```python
from build123d import *

# Parameters (mm, degrees)
F0_R      = 1.1
F1_DEPTH  = 4.75
F2_R      = 5
F3_DEPTH  = 5
F5_R      = 2
F7_DEPTH  = 0.8
F8_R      = 0.75
F9_R      = 9.5
F10_DEPTH = 3
F12_R     = 4.5172071506
F12_R_2   = 2.2672071506
F13_DEPTH = 3.7
F14_R     = 0.625
F15_DEPTH = 2
F16_SIZE  = 0.35


# Not quite as in the source:
# - a feature names something its author has since deleted; it is built from what else it names


with BuildPart() as f1:
    # F0 (on Top) → F1 (new body)
    with BuildSketch(Plane.XY):
        with BuildLine():
            Line((-5.0334316447, -3.2656646917), (-9.6784130262, -7.9106460732))
            ThreePointArc((-9.6784130262, -7.9106460732), (-7.1490584463, -10.2538267653), (-4.0757746589, -11.8168549509))
            ThreePointArc((-4.0757746589, -11.8168549509), (-3.593311946, -12.8676823003), (-2.8459674038, -13.75))
            Line((-2.8459674038, -13.75), (2.8459674038, -13.75))
            ThreePointArc((2.8459674038, -13.75), (3.593311946, -12.8676823003), (4.0757746589, -11.8168549509))
            ThreePointArc((4.0757746589, -11.8168549509), (7.1490584463, -10.2538267653), (9.6784130262, -7.9106460732))
            Line((9.6784130262, -7.9106460732), (5.0334316447, -3.2656646917))
            ThreePointArc((5.0334316447, -3.2656646917), (0, 6), (-5.0334316447, -3.2656646917))
        make_face()
        with Locations((0, -11.25)):
            Circle(F0_R, mode=Mode.SUBTRACT)
        with BuildLine():
            Line((-5.061459087, -6.82922604), (-3.2656646917, -5.0334316447))
            ThreePointArc((-3.2656646917, -5.0334316447), (0, -6), (3.2656646917, -5.0334316447))
            Line((3.2656646917, -5.0334316447), (5.061459087, -6.82922604))
            ThreePointArc((5.061459087, -6.82922604), (4.8326547168, -8.5179809488), (3.2656646917, -7.8480653995))
            ThreePointArc((3.2656646917, -7.8480653995), (0, -8.5003938964), (-3.2656646917, -7.8480653995))
            ThreePointArc((-3.2656646917, -7.8480653995), (-4.8326547168, -8.5179809488), (-5.061459087, -6.82922604))
        make_face(mode=Mode.SUBTRACT)
    extrude(amount=F1_DEPTH)

    # F2 (on face) → F3 (join)
    with BuildSketch(Plane.XY.offset(4.75)):
        Circle(F2_R)
    extrude(amount=F3_DEPTH)

    # F5
    f5_edges = [f1.edges().sort_by_distance(p)[0] for p in [
        (3.265665, -7.848065, 2.375),
        (-3.265665, -7.848065, 2.375),
        (-9.678413, -7.910646, 2.375),
        (-4.075775, -11.816855, 2.375),
        (9.678413, -7.910646, 2.375),
        (4.075775, -11.816855, 2.375),
    ]]
    fillet(f5_edges, radius=F5_R)

    # F6 (on face) → F7 (cut)
    with BuildSketch(Plane.XY.offset(4.75)):
        Polygon((4.3772207939, -8.619861481), (8.619861481, -4.3772207939), (6.2942457002, -2.1069760406), (2.0792905268, -6.3219312139), align=None)
        Polygon((-4.3772207939, -8.619861481), (-2.0792905268, -6.3219312139), (-6.2942457002, -2.1069760406), (-8.619861481, -4.3772207939), align=None)
    extrude(amount=-F7_DEPTH, mode=Mode.SUBTRACT)

    # F8
    f8_edges = [f1.edges().sort_by_distance(p)[0] for p in [
        (4.200611, -4.200611, 3.95),
        (-4.200611, -4.200611, 3.95),
        (-5, 0, 4.75),
        (-5, 0, 9.75),
        (6.378475, -6.618607, 3.95),
        (-6.378475, -6.618607, 3.95),
    ]]
    fillet(f8_edges, radius=F8_R)

    # F9 (on Top) → F10 (cut)
    with BuildSketch(Plane.XY):
        Circle(F9_R)
    extrude(amount=F10_DEPTH, mode=Mode.SUBTRACT)

    # F12 (on face) → F13 (cut)
    with BuildSketch(Plane(origin=(0, 0, 3), x_dir=(1, 0, 0), z_dir=(0, 0, -1))):
        Circle(F12_R)
        Circle(F12_R_2, mode=Mode.SUBTRACT)
    extrude(amount=-F13_DEPTH, mode=Mode.SUBTRACT)

    # F14 (on face) → F15 (join)
    with BuildSketch(Plane(origin=(0, 0, 0), x_dir=(1, 0, 0), z_dir=(0, 0, -1))):
        with Locations((7.6240489866, 8.007460935)):
            Circle(F14_R)
        with Locations((-7.6240489866, 8.007460935)):
            Circle(F14_R)
    extrude(amount=F15_DEPTH)

    # F16
    f16_edges = [f1.edges().sort_by_distance(p)[0] for p in [
        (6.999049, -8.007461, -2),
        (-8.249049, -8.007461, -2),
    ]]
    chamfer(f16_edges, length=F16_SIZE)


solid = f1.part
```
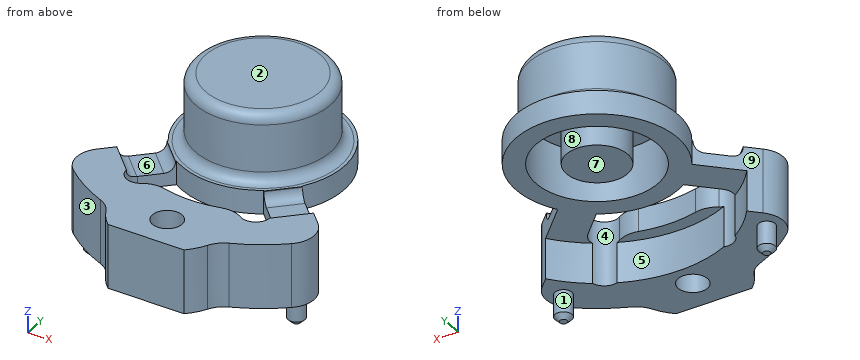
Input: part model. Units: mm. Frame: model coordinates. Face numbers are marked on the shaded views. A direction names the side the tool comes from. Give positions to 0.01 mm unless a question says otherwise; leave off trailing zeros. Write each loop counter-clockwise with the first axis right and the second up, starting at its lowest first coordinate (ties: lowest second). Pieces come first, ordered by that corner, then holes. Notation, with made-up numbers: (18, 38.5) - (69, 38.5) arc R24 ccw to (69, 48.5) - close; hole circle Ø2 at (72, -27). An arc over 180 degrees is marked (long way). Write item = value, one per line. Start each with the question number.
1. Mould query, pull axis X, two halves, no side actions, for the marked faces 1, 2, 3 and 4. Classes: released by +X, released by -X, zero draft, split by the parting line, or undercut.
2. Section query C-C, the plane z = 8.75. Output: boundary loops of the cut face in (x, y).
3. Section query A-A, the plane x = 0. Count the separate pieces of the cut face and the enclosed holes in it, then the cut area to 3 significant figures.
4. Ray query, L1, parallel to Y at x = 0, z = 5.15; L2, parallel to Y at x = 0, z = 4.5; L3, parallel to X at y = 0, z = 4.4. Return the intervals inside material, ascending.
5. Section query B-B, the plane y = -11.25. Output: boundary loops of the cut face in (x, z).
6. Section query D-D, the plane y = 0. Output: boundary loops of the cut face in (x, z), then the cut area to 4 significant figures.
7. First-contact query: pin 1 Ø10 at (x, y) = (-2, -1.5) entering from -Z; pin 2 Ø2.5 at (x, y) = (-5, -6) entering from +Z; pin 3 Ø3 at (x, y) = (0, -11.25) entering from -Z. Flat tips, straight axial feed; report the tip coordinate or a pass-through.
8. Access query for the marked faces 5, 6, 7, 8 and 9. Directions: +Z, -Z, +X, -X, +Y, -Y. A direction counts if a zero-diameter tool reaches every point of the face in a straight line with its end or side. Return the directions, or none.
Check sheet entries:
q1.face_1 = undercut
q1.face_2 = zero draft
q1.face_3 = released by -X
q1.face_4 = undercut
q2.outline = circle Ø10 at (0, 0)
q3.separate_pieces = 3
q3.enclosed_holes = 0
q3.area = 65.8 mm2
q4.L1 = -5.09 to -4.52, -2.27 to 2.27, 4.52 to 5.09
q4.L2 = -13.75 to -12.35, -10.15 to -8.5, -6 to -4.52, -2.27 to 2.27, 4.52 to 6
q4.L3 = -6 to -4.52, -2.27 to 2.27, 4.52 to 6
q5.outline = (-5.45, 0) - (-1.1, 0) - (-1.1, 4.75) - (-5.45, 4.75) - close; (1.1, 0) - (5.45, 0) - (5.45, 4.75) - (1.1, 4.75) - close
q6.outline = (-6, 3) - (-4.52, 3) - (-4.52, 6.7) - (-2.27, 6.7) - (-2.27, 3) - (2.27, 3) - (2.27, 6.7) - (4.52, 6.7) - (4.52, 3) - (6, 3) - (6, 4.75) - (5.75, 4.75) arc R0.75 cw to (5, 5.5) - (5, 9) arc R0.75 ccw to (4.25, 9.75) - (-4.25, 9.75) arc R0.75 ccw to (-5, 9) - (-5, 5.5) arc R0.75 cw to (-5.75, 4.75) - (-6, 4.75) - close
q6.area = 54.35 mm2
q7.pin_1 = 3
q7.pin_2 = 4.23
q7.pin_3 = 0
q8.face_5 = -Z, +Y
q8.face_6 = +Z
q8.face_7 = -Z, +X, -X, +Y
q8.face_8 = -Z
q8.face_9 = +Z, -Z, -X
